```python
from build123d import *

# Parameters (mm, degrees)
ESQUISSE1_R                = 10
BOSS_EXTRU_1_DEPTH         = 83
ESQUISSE2_R                = 6
BOSS_EXTRU_2_DEPTH         = 1.5
ESQUISSE5_R                = 3
ENL_V_MAT_EXTRU_2_DEPTH    = 25
ESQUISSE9_W                = 1.25
ESQUISSE9_H                = 10
ESQUISSE18_W               = 2.1
ESQUISSE18_H               = 10
TROU_TARAUD_M53_AT_2_COUNT = 2
TROU_TARAUD_M53_AT_2_PITCH = 20
ESQUISSE19_R               = 2.5
ENL_V_MAT_EXTRU_3_DEPTH    = 86.675259097


with BuildPart() as part:
    # Esquisse1 → Boss.-Extru.1 (new body)
    with BuildSketch(Plane(origin=(0, 0, 0), x_dir=(0, 0, -1), z_dir=(1, 0, 0))):
        Circle(ESQUISSE1_R)
    extrude(amount=BOSS_EXTRU_1_DEPTH)

    # Esquisse2 → Boss.-Extru.2 (add)
    with BuildSketch(Plane(origin=(83, 0, 0), x_dir=(0, 0, -1), z_dir=(1, 0, 0))):
        Circle(ESQUISSE2_R)
    extrude(amount=BOSS_EXTRU_2_DEPTH)

    # Esquisse5 → Enlèv. mat.-Extru.2 (cut)
    with BuildSketch(Plane(origin=(84.5, 0, 0), x_dir=(0, 0, -1), z_dir=(1, 0, 0))):
        Circle(ESQUISSE5_R)
    extrude(amount=-ENL_V_MAT_EXTRU_2_DEPTH, mode=Mode.SUBTRACT)

    # Esquisse9 → Trou taraudé M31 (revolve, cut)
    with BuildSketch(Plane(origin=(78, 0, 0), x_dir=(0, 0, -1), z_dir=(1, 0, 0))):
        with Locations((0.625, 5)):
            Rectangle(ESQUISSE9_W, ESQUISSE9_H)
    revolve(axis=Axis((78, -6.35, 0), (0, 1, 0)), mode=Mode.SUBTRACT)

    # Esquisse18 → Trou taraudé M53 (revolve, cut)
    with BuildSketch(Plane(origin=(10, 0, 0), x_dir=(0, 0, -1), z_dir=(1, 0, 0))):
        with Locations((1.05, 5)):
            Rectangle(ESQUISSE18_W, ESQUISSE18_H)
    trou_taraud_m53 = revolve(axis=Axis((10, -6.35, 0), (0, 1, 0)), mode=Mode.SUBTRACT)

    # Trou taraudé M53 at 2: Trou taraudé M53 ×2
    with Locations(*[(i * TROU_TARAUD_M53_AT_2_PITCH, 0, 0) for i in range(1, TROU_TARAUD_M53_AT_2_COUNT)]):
        add(trou_taraud_m53, mode=Mode.SUBTRACT)

    # Esquisse19 → Enlèv. mat.-Extru.3 (cut, through all)
    with BuildSketch(Plane(origin=(0, 0, 0), x_dir=(1, 0, 0), z_dir=(0, 1, 0))):
        with Locations(Location((10, 0, 0), (0, 0, 270))):
            Circle(ESQUISSE19_R)
        with Locations(Location((30, 0, 0), (0, 0, 270))):
            Circle(ESQUISSE19_R)
    extrude(amount=-ENL_V_MAT_EXTRU_3_DEPTH, mode=Mode.SUBTRACT)


solid = part.part
```
Model file for the job. Use its own axes, mm. A direction names the side the tool comes from. Give positions to 0.01 mm unless a question says otherwise; leave off trailing zeros. Loops run counter-clockwise (first coordinate to the right, second up) from the corner with the lowest first, then second, coordinate; pieces in that order, holes last. Notation, with made-up numbers: M -38.75,-22 L -28.75,-22 A26 cw -28.75,2 Z; hole C 23,-38 d3. An arc over 180 degrees is marked long. Use one line per item in the form item = value.
Item 1: Two-plate mould, pull along X, no slides. Class faces 6 (the cylindrical face through (32.05, 5.07, 0.46)), 7 (the cylindrical face through (7.56, -4.93, -0.54)), 8 (the cylindrical face through (72.18, -2.93, 0.65)), 9 (the flat face through (59.5, 0, 0)): released by +X, released by -X, zero draft, split by the parting line, or undercut.
Filled in:
face_6 = undercut
face_7 = undercut
face_8 = zero draft
face_9 = released by +X
Item 2: Slice it at C-C on y = -7.75. List the corners of the cut face in (x, z), and give its area (3 significant figures).
Filled in:
outline = M 0,-6.32 L 83,-6.32 L 83,6.32 L 0,6.32 Z; hole C 10,0 d5; hole C 30,0 d5
area = 1,010 mm^2
Item 3: Slice it at A-A on z = 0. Give the number of separate pieces and of enclosed holes in the cut face, and give its area (3 significant figures).
Filled in:
separate_pieces = 4
enclosed_holes = 0
area = 1,330 mm^2
Item 4: Drill centre lines: L1, parallel to X at y = -7.75, z = 0; L2, parallel to X at y = 6.25, z = 0; L3, parallel to X at y = 3.5, z = 1.75. Where is each one in solid material? Low to high.
Filled in:
L1 = 0 to 7.5, 12.5 to 27.5, 32.5 to 83
L2 = 0 to 7.9, 12.1 to 27.9, 32.1 to 76.75, 79.25 to 83
L3 = 0 to 8.84, 11.16 to 28.84, 31.16 to 84.5
Item 5: Flat gauge pins, fed straight in: pin 1 Ø5 at (y, z) = (0, 0) entering from +X; pin 2 Ø3 at (x, y) = (46.5, -5) entering from -Z; pin 3 Ø3 at (x, y) = (9.5, -3.5) entering from +Z. Where does each tip first touch, or does it go through?
Filled in:
pin_1 = 59.5
pin_2 = -9.37
pin_3 = 9.8
Item 6: Slice it at D-D on x = 47. List the corners of the cut face in (y, z).
Filled in:
outline = C 0,0 d20
Item 7: Slice it at B-B on x = 10. List the corners of the cut face in (y, z), and give its area (3 significant figures).
Filled in:
outline = M -9.68,-2.5 A10 ccw 9.78,-2.1 L 0,-2.1 L 0,-2.5 Z; M -9.68,2.5 L 0,2.5 L 0,2.1 L 9.78,2.1 A10 ccw Z
area = 223 mm^2
Item 8: Which spindle directions (+Z, -Z, +X, -X, +Y, -Y) get a long thin tool onto all of the face, cutting with end or side? Do faces 1 (the cylindrical face through (7.918, 5.07, 0.273)), 2 (the cylindrical face through (32.11, -4.93, 1.34)), 3 (the cylindrical face through (76.76, 6.41, 0.16)), 4 (the cylindrical face through (40.92, -9.76, 2.17)), 5 (the flat face through (83, -7, 0)). Say none if no direction does.
Filled in:
face_1 = +Y, -Y
face_2 = -Y
face_3 = +Y
face_4 = +X, -X
face_5 = +X
